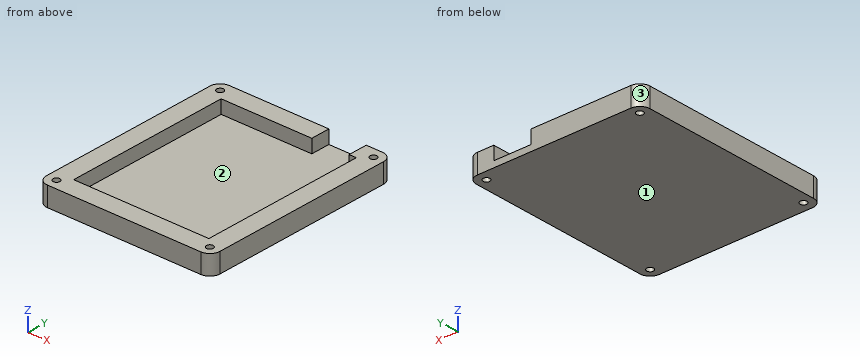
```python
from build123d import *

# Parameters (mm, degrees)
SKETCH_W        = 86
SKETCH_H        = 101
PAD_DEPTH       = 3
SKETCH001_W     = 86
SKETCH001_H     = 101
SKETCH001_W_2   = 67
SKETCH001_H_2   = 82
PAD001_DEPTH    = 6.6
SKETCH002_R     = 1.7
POCKET_DEPTH    = 12
SKETCH003_W     = 18.5
SKETCH003_H     = 9.5
POCKET001_DEPTH = 6.6
FILLET_R        = 5


with BuildPart() as part:
    # Sketch → Pad (new body)
    with BuildSketch(Plane.XY):
        Rectangle(SKETCH_W, SKETCH_H)
    extrude(amount=PAD_DEPTH)

    # Sketch001 (on Face6 of Pad) → Pad001 (join)
    with BuildSketch(Plane.XY.offset(3)):
        Rectangle(SKETCH001_W, SKETCH001_H)
        Rectangle(SKETCH001_W_2, SKETCH001_H_2, mode=Mode.SUBTRACT)
    extrude(amount=PAD001_DEPTH)

    # Sketch002 (on Face3 of Pad001) → Pocket (cut)
    with BuildSketch(Plane.XY.offset(9.6)):
        with Locations((-38, -45.5)):
            Circle(SKETCH002_R)
        with Locations((-38, 45.5)):
            Circle(SKETCH002_R)
        with Locations((38, 45.5)):
            Circle(SKETCH002_R)
        with Locations((38, -45.5)):
            Circle(SKETCH002_R)
    extrude(amount=-POCKET_DEPTH, mode=Mode.SUBTRACT)

    # Sketch003 (on Face10 of Pocket) → Pocket001 (cut)
    with BuildSketch(Plane.XY.offset(9.6)):
        with Locations((20.676, 45.75)):
            Rectangle(SKETCH003_W, SKETCH003_H)
    extrude(amount=-POCKET001_DEPTH, mode=Mode.SUBTRACT)

    # Fillet
    fillet_edges = [part.edges().sort_by_distance(p)[0] for p in [
        (43, -50.5, 4.8),
        (-43, -50.5, 4.8),
        (-43, 50.5, 4.8),
        (43, 50.5, 4.8),
    ]]
    fillet(fillet_edges, radius=FILLET_R)


solid = part.part
```
Here's how the part is built. I have some questions about the finished solid (model axes, mm). Face numbers are marked on the shaded views. Give positions to 0.01 mm unless a question says otherwise; leave off trailing zeros. Loops run counter-clockwise (first coordinate to the right, second up) from the corner with the lowest first, then second, coordinate; pieces in that order, holes last. Notation, with made-up numbers: (42.25, 88) -> (91.25, 88) arc R30 ccw to (91.25, 123) -> close; hole circle Ø8 at (-10.75, 26.25). An arc over 180 degrees is marked (long way). Use one line per item in the form item = value. Start each with the question number.
1) Thinking about a two-plate mould opening in X: for the marked faces 1, 2 and 3, which applies, +X half, -X half, draft (parallel to the pull), parting line (faces both ways), or undercut?
2) Imagine slicing it at B-B (y = 25.5). Please give me the cut outline in (x, z), then the cut area to 3 significant figures.
3) Imagine slicing it at A-A (z = 4.75). Please give me the cut outline in (x, y), then the cut area to 3 significant figures.
4) For P1, Ø1.5, axis at x = -7.5, y = 33, coming from the +Z side; P2, Ø4.5, axis at x = 38, y = -45.5, coming from the +Z side, each with a flat end and sliding along its axis, tell me the tip position at first contact or that it passes through.
5) Please list where these lines run through material, in increasing order: line 1 along Y through (x, z) = (38, 6.75); line 2 along X through (y, z) = (12, 5); line 3 along Y through (x, z) = (37.5, 7).
6) Imagine slicing it at C-C (x = -13). Please give me the cut outline in (y, z), then the cut area to 3 significant figures.
7) Imagine slicing it at D-D (x = 22.5). Please give me the cut outline in (y, z), then the cut area to 3 significant figures.
Check values:
q1.face_1 = draft
q1.face_2 = undercut
q1.face_3 = -X half
q2.outline = (-43, 0) -> (43, 0) -> (43, 9.6) -> (33.5, 9.6) -> (33.5, 3) -> (-33.5, 3) -> (-33.5, 9.6) -> (-43, 9.6) -> close
q2.area = 383 mm^2
q3.outline = (-43, -45.5) arc R5 ccw to (-38, -50.5) -> (38, -50.5) arc R5 ccw to (43, -45.5) -> (43, 45.5) arc R5 ccw to (38, 50.5) -> (29.93, 50.5) -> (29.93, 41) -> (33.5, 41) -> (33.5, -41) -> (-33.5, -41) -> (-33.5, 41) -> (11.43, 41) -> (11.43, 50.5) -> (-38, 50.5) arc R5 ccw to (-43, 45.5) -> close; hole circle Ø3.4 at (-38, -45.5); hole circle Ø3.4 at (-38, 45.5); hole circle Ø3.4 at (38, -45.5); hole circle Ø3.4 at (38, 45.5)
q3.area = 2,960 mm^2
q4.P1 = 3
q4.P2 = 9.6
q5.line_1 = -50.5 to -47.2, -43.8 to 43.8, 47.2 to 50.5
q5.line_2 = -43 to -33.5, 33.5 to 43
q5.line_3 = -50.5 to -47.12, -43.88 to 43.88, 47.12 to 50.5
q6.outline = (-50.5, 0) -> (50.5, 0) -> (50.5, 9.6) -> (41, 9.6) -> (41, 3) -> (-41, 3) -> (-41, 9.6) -> (-50.5, 9.6) -> close
q6.area = 428 mm^2
q7.outline = (-50.5, 0) -> (50.5, 0) -> (50.5, 3) -> (-41, 3) -> (-41, 9.6) -> (-50.5, 9.6) -> close
q7.area = 366 mm^2
